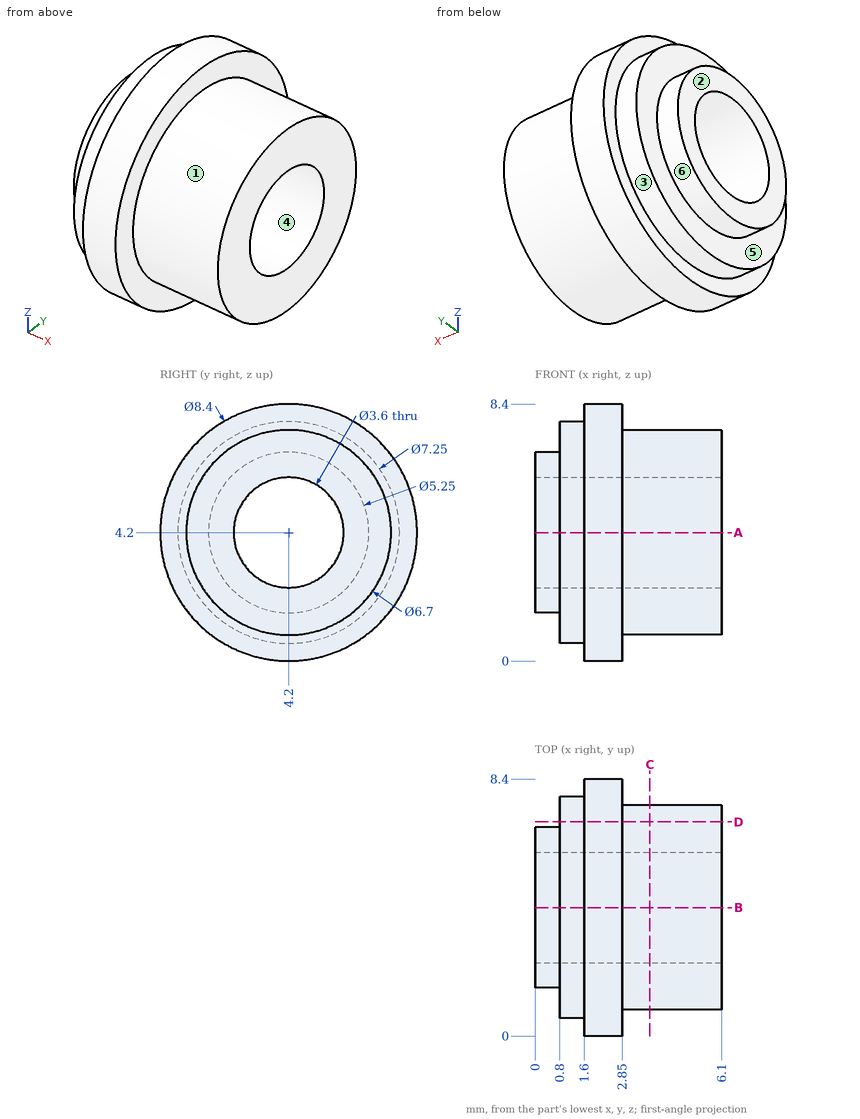
Here's the drawing with two shaded views (mm, measured from the low corner). I have some questions. A direction names the side the tool comes from. Coordinates: 2 decimals unless noted, no trailing zeros. Order: outer loops, then holes, each group sorted by start corner. A loop starts at its lowest first (then second) coordinate and runs counter-clockwise, first axis right, second up. Notation, with made-up numbers: (56, 44.25) - (82, 44.25) arc R22 cw to (82, 77.25) - close; hole circle Ø9 at (-16, -35). An arc over 180 degrees is marked (long way). Answer in a Markdown table with one row per item.
1. For the marked faces 1, 2 and 3, which set-ups out of +Z, -Z, +X, -X, +Y, -Y let a thin tool reach every point of the face, with its end or its side?
Reply:
| item | result |
|---|---|
| face 1 | +X |
| face 2 | +Z, -Z, -X, +Y, -Y |
| face 3 | -X |
2. If I drill on line 1 along Y through (x, z) = (3.5, 4.25); line 2 along Z through (x, y) = (1.5, 4.2) (3 decimals); line 3 along Z through (x, y) = (2, 4.2), over which ranges is the centre line in solid material (lowest first)?
Reply:
| item | result |
|---|---|
| line 1 | y = 0.85 to 2.4, 6 to 7.55 |
| line 2 | z = 0.575 to 2.4, 6 to 7.825 |
| line 3 | z = 0 to 2.4, 6 to 8.4 |
3. For pin 1 (4 mm diameter, centred on y = 5, z = 5, fed in from +X); pin 2 (1 mm diameter, centred on y = 1, z = 2, fed in from -X); pin 3 (1 mm diameter, centred on x = 4, y = 7.5, fed in from -Z), each with a flat end and sliding along its axis, tell me the tip position at first contact or that it passes through.
Reply:
| item | result |
|---|---|
| pin 1 | stops at x = 6.1 |
| pin 2 | stops at x = 0.8 |
| pin 3 | stops at z = 2.36 |
4. Suppose I cut it at D-D (y = 7). Please give me the cut outline in (x, z).
Reply:
| item | result |
|---|---|
| outline | (0.8, 1.9) - (1.6, 1.9) - (1.6, 1.07) - (2.85, 1.07) - (2.85, 2.36) - (6.1, 2.36) - (6.1, 6.04) - (2.85, 6.04) - (2.85, 7.33) - (1.6, 7.33) - (1.6, 6.5) - (0.8, 6.5) - close |
5. Suppose I cut it at A-A (z = 4.2). Please give me the cut outline in (x, y) (3 decimals).
Reply:
| item | result |
|---|---|
| outline | (0, 1.575) - (0.8, 1.575) - (0.8, 0.575) - (1.6, 0.575) - (1.6, 0) - (2.85, 0) - (2.85, 0.85) - (6.1, 0.85) - (6.1, 2.4) - (0, 2.4) - close; (0, 6) - (6.1, 6) - (6.1, 7.55) - (2.85, 7.55) - (2.85, 8.4) - (1.6, 8.4) - (1.6, 7.825) - (0.8, 7.825) - (0.8, 6.825) - (0, 6.825) - close |
6. Suppose I cut it at C-C (x = 3.75). Please give me the cut outline in (y, z).
Reply:
| item | result |
|---|---|
| outline | circle Ø6.7 at (4.2, 4.2); hole circle Ø3.6 at (4.2, 4.2) |
7. If we mould it in two halves opening along Z, with no side actions, what happens to the marked faces 4, 5 and 6? For each: pulls with the +Z half, pulls with the -Z half, needs draft (parallel to the pull), parting line crosses it, or undercut.
Reply:
| item | result |
|---|---|
| face 4 | undercut |
| face 5 | needs draft |
| face 6 | parting line crosses it |
